Input: dimensioned drawing with shaded views. Units: mm. Origin: part minimum x, y, z. Round coordinates to 2 decimals unless told otherwise and drop trailing zeros. Order: outer loops, then holes, each group sorted by start corner. A loop starts at its lowest first (then second) coordinate and runs counter-clockwise, first axis right, second up.
Item 1: Line query: L1, parallel to Y at x = 28, z = 0.85; L2, parallel to X at y = 11, z = 1.05 (1 decimal). Output: solid intervals per line, ascending.
Item 2: Cut plane D-D on z = 0.9. Give the number of separate pieces and of enclosed holes in the cut face.
Item 3: Cut plane C-C on x = 30. Output: boundary loops of the cut face in (y, z).
Item 4: First-contact query: pin 1 (19 mm diameter, centred on x = 19, y = 19, fed in from +Z); pin 2 (1.8 mm diameter, centred on x = 26.78, y = 11.22, fed in from +Z). Flat tips, straight axial feed; report the tip coordinate or a pass-through.
Item 5: Cut plane A-A on y = 19. Output: boundary loops of the cut face in (x, z), then the cut area to 3 significant figures.
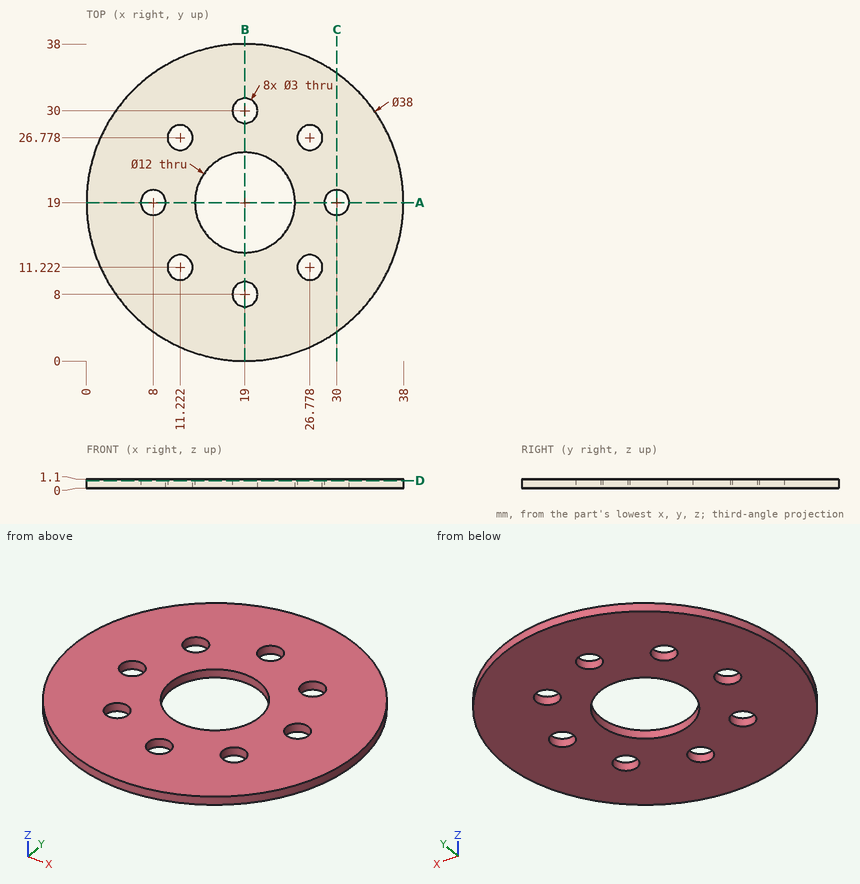
From the geometry:
1. L1: y = 2.27 to 10.35, 12.09 to 25.91, 27.65 to 35.73
1. L2: x = 1.8 to 9.7, 12.7 to 25.3, 28.3 to 36.2
2. separate pieces: 1
2. enclosed holes: 9
3. outline: (3.51, 0) - (17.5, 0) - (17.5, 1.1) - (3.51, 1.1) - close; (20.5, 0) - (34.49, 0) - (34.49, 1.1) - (20.5, 1.1) - close
4. pin 1: stops at z = 1.1
4. pin 2: passes through
5. outline: (0, 0) - (6.5, 0) - (6.5, 1.1) - (0, 1.1) - close; (9.5, 0) - (13, 0) - (13, 1.1) - (9.5, 1.1) - close; (25, 0) - (28.5, 0) - (28.5, 1.1) - (25, 1.1) - close; (31.5, 0) - (38, 0) - (38, 1.1) - (31.5, 1.1) - close
5. area: 22.0 mm2
